Verification items for the finished model (mm, model axes). A direction names the side the tool comes from. Round coordinates to 2 decimals unless told otherwise and drop trailing zeros. Loops run counter-clockwise (first coordinate to the right, second up) from the corner with the lowest first, then second, coordinate; pieces in that order, holes last. Notation, with made-up numbers: M 63.5,89 L 110.5,89 A20 ccw 110.5,116 Z; hole C 6,81.5 d1. An arc over 180 degrees is marked long. Answer as CSV lines item,"result".
```python
from build123d import *

# Parameters (mm, degrees)
F0_R      = 7.62
F0_R_2    = 5.55625
F1_DEPTH  = 11.4935
F3_W      = 19.05
F3_H      = 19.05
F3_R      = 5.55625
F4_DEPTH  = 2.54
F6_W      = 19.05
F6_H      = 19.05
F6_R      = 5.55625
F7_DEPTH  = 0.79375
F9_W      = 19.05
F9_H      = 19.05
F9_R      = 5.55625
F10_DEPTH = 0.79375
F12_W     = 19.05
F12_H     = 19.05
F12_R     = 5.55625
F13_DEPTH = 3.302
F15_D     = 1.999996
F15_DEPTH = 3.302
F16_R     = 1.0922
F17_DEPTH = 2.54
F19_DEPTH = 11.43
F21_DEPTH = 11.43


with BuildPart() as f1:
    # F0 (on Top) → F1 (new body, symmetric)
    with BuildSketch(Plane.XY):
        Circle(F0_R)
        Circle(F0_R_2, mode=Mode.SUBTRACT)
    extrude(amount=F1_DEPTH, both=True)

    # F3 (on offset) → F4 (join)
    with BuildSketch(Plane(origin=(0, 0, -10.6045), x_dir=(1, 0, 0), z_dir=(0, 0, -1))):
        Rectangle(F3_W, F3_H)
        Circle(F3_R, mode=Mode.SUBTRACT)
    extrude(amount=-F4_DEPTH)

    # F6 (on offset) → F7 (join)
    with BuildSketch(Plane(origin=(0, 0, 3.3655), x_dir=(1, 0, 0), z_dir=(0, 0, -1))):
        Rectangle(F6_W, F6_H)
        Circle(F6_R, mode=Mode.SUBTRACT)
    extrude(amount=-F7_DEPTH)

    # F9 (on offset) → F10 (join)
    with BuildSketch(Plane(origin=(0, 0, 5.0165), x_dir=(1, 0, 0), z_dir=(0, 0, -1))):
        Rectangle(F9_W, F9_H)
        Circle(F9_R, mode=Mode.SUBTRACT)
    extrude(amount=-F10_DEPTH)

    # F12 (on offset) → F13 (join)
    with BuildSketch(Plane(origin=(0, 0, 7.3025), x_dir=(1, 0, 0), z_dir=(0, 0, -1))):
        Rectangle(F12_W, F12_H)
        Circle(F12_R, mode=Mode.SUBTRACT)
    extrude(amount=-F13_DEPTH)

    # F15
    with Locations(Plane.XY.offset(10.6045)):
        with Locations((-6.477, -6.477), (-6.477, 6.477), (6.477, 6.477), (6.477, -6.477)):
            Hole(F15_D / 2, depth=F15_DEPTH)

    # F16 (on face) → F17 (cut, through all)
    with BuildSketch(Plane(origin=(0, 0, -10.6045), x_dir=(1, 0, 0), z_dir=(0, 0, -1))):
        with Locations((-7.874, 6.985)):
            Circle(F16_R)
        with Locations((7.747, 7.207488)):
            Circle(F16_R)
        with Locations((7.747, -7.207488)):
            Circle(F16_R)
        with Locations((-7.874, -6.985)):
            Circle(F16_R)
    extrude(amount=-F17_DEPTH, mode=Mode.SUBTRACT)

    # F18 (on face) → F19 (cut)
    with BuildSketch(Plane(origin=(0, 0, -11.4935), x_dir=(1, 0, 0), z_dir=(0, 0, -1))):
        with BuildLine():
            ThreePointArc((2.54519, 4.93902), (1.723461, 6.558707), (0, 7.131685))
            ThreePointArc((0, 7.131685), (-1.723461, 6.558707), (-2.54519, 4.93902))
            ThreePointArc((-2.54519, 4.93902), (0, 5.55625), (2.54519, 4.93902))
        make_face()
    extrude(amount=-F19_DEPTH, mode=Mode.SUBTRACT)

    # F20 (on Front) → F21 (cut)
    with BuildSketch(Plane.XZ):
        with BuildLine():
            Line((1.9812, 2.3368), (-1.9812, 2.3368))
            ThreePointArc((-1.9812, 2.3368), (-3.5687, 0.7493), (-1.9812, -0.8382))
            Line((-1.9812, -0.8382), (1.9812, -0.8382))
            ThreePointArc((1.9812, -0.8382), (3.5687, 0.7493), (1.9812, 2.3368))
        make_face()
    extrude(amount=F21_DEPTH, mode=Mode.SUBTRACT)


solid = f1.part
```
1) Material ranges on probe 1 along Z at (x, y) = (6.5, -7.25); probe 2 along Z at (x, y) = (8.25, -6.75); probe 3 along Z at (x, y) = (-7, 4.25), recorded low to high.
Here are the results:
probe 1,"z = -10.6 to -8.06, 3.37 to 4.16, 5.02 to 5.81"
probe 2,"z = 3.37 to 4.16, 5.02 to 5.81, 7.3 to 10.6"
probe 3,"z = -10.6 to -8.06, 3.37 to 4.16, 5.02 to 5.81, 7.3 to 10.6"
2) Section check B-B (z = -2.75). Record the cut outline in (x, y).
Here are the results:
outline,"C 0,0 d15.24; hole M -2.55,-4.94 A2.39 ccw 0,-7.13 A2.39 ccw 2.55,-4.94 A5.56 ccw long Z"
3) Draft check along X on faces 5 (the flat face through (0, 9.525, 9)), 6 (the flat face through (0, -7.4, -0.838)), 7 (the flat face through (-9.525, 0, -9)). Enter one of: +X half, -X half, draft (parallel to the pull), parting line (faces both ways), or undercut.
Here are the results:
face 5,"draft"
face 6,"undercut"
face 7,"-X half"
4) Section check A-A (x = -1.5). State how many separate pieces and enclosed holes the cut face has, plus the area to 3 significant figures.
Here are the results:
separate pieces,"3"
enclosed holes,"0"
area,"107 mm^2"
5) Go/stop test with flat-tipped pins: pin 1 (3 mm diameter, centred on x = 7.75, y = 7.21, fed in from +Z); pin 2 (1.8 mm diameter, centred on x = -6.477, y = -6.477, fed in from -Z); pin 3 (1.2 mm diameter, centred on x = -6.477, y = 6.477, fed in from +Z); pin 4 (5.5 mm diameter, centred on x = 2, y = -0.5, fed in from +Z). Record where each tip stops, or that it passes through.
Here are the results:
pin 1,"stops at z = 10.6"
pin 2,"stops at z = -10.6"
pin 3,"stops at z = 5.81"
pin 4,"passes through"
6) Set-up check for faces 1 (the cylindrical face through (-1.65, -7.44, 11.06)), 2 (the flat face through (-6.5, -4.4, 5.016)), 3 (the cylindrical face through (-3.57, -5.79, 0.78)), 4 (the cylindrical face through (7.605, 6.125, -9.352)): record each of +Z, -Z, +X, -X, +Y, -Y from which the full face is reachable in a straight line by a thin tool's end or side.
Here are the results:
face 1,"+Z"
face 2,"none"
face 3,"-Y"
face 4,"-Z"
